The model under review builds one solid part; all positions refer to its coordinate system, in mm. A direction names the side the tool comes from. Coordinates: 2 decimals unless noted, no trailing zeros. Write each loop counter-clockwise with the first axis right and the second up, starting at its lowest first coordinate (ties: lowest second). Pieces come first, ordered by that corner, then holes.
1) Machinability: for faces 5 (the flat face through (137, 6, -5)), 6 (the flat face through (16, 0, -60)), which of the approach directions +Z, -Z, +X, -X, +Y, -Y give a long, thin tool a straight path to every point of the face, cutting with its end or side? Answer none if there is none.
2) For line 1 (Z direction, x = 287.5, y = 3.8); line 2 (Z direction, x = 385.5, y = 3.8); line 3 (X direction, y = -1, z = -129.5), list the stretches that pass through material, from the lowest coordinate up.
3) Add section C-C, the plane z = -29. State the section outline as (x, y) points.
4) Mouldability with a two-part tool opening along X and no side actions: class faces 1 (the flat face through (0, -2, -81)), 2 (the flat face through (390.8, -2, -81)), 3 (the cylindrical face through (10.12, -10.86, -108)), 4 (the cylindrical face through (380.757, -0.487, -9.349)) as released by +X, released by -X, zero draft, split by the parting line, or undercut.
5) For P1, Ø3, axis at x = 195.41, z = -129.5, coming from the -Y side; P2, Ø6, axis at x = 197, z = -15, coming from the -Y side; P3, Ø4, axis at x = 242.5, y = -9.5, coming from the -Z side, all flat-tipped, find the tip position at first contact; note any pin that passes through.
6) Add section B-B, the plane z = -78. State the section outline as (x, y) points, then the cut area to 3 significant figures.
7) Add section A-A, the plane x = 365. State the section outline as (y, z) points.
from build123d import *

# Parameters (mm, degrees)
SKETCH1_W               = 390.8
SKETCH1_H               = 133.8
BOSS_EXTRUDE1_DEPTH     = 6
SKETCH2_W               = 370.8
SKETCH2_H               = 125.6
CUT_EXTRUDE1_DEPTH      = 4
BOSS_EXTRUDE3_DEPTH     = 390.8
BOSS_EXTRUDE4_DEPTH     = 4
CUT_EXTRUDE6_DEPTH      = 414.309625425
CUT_EXTRUDE6_DEPTH_BACK = 414.309625425
SKETCH15_R              = 5
CUT_EXTRUDE8_DEPTH      = 1
SKETCH16_W              = 12.5
SKETCH16_H              = 19.4
CUT_EXTRUDE9_DEPTH      = 6
SKETCH17_W              = 390.8
SKETCH17_H              = 133.8
SKETCH17_W_2            = 386.8
SKETCH17_H_2            = 129.8
CUT_EXTRUDE10_DEPTH     = 1.7
SKETCH18_W              = 370.8
SKETCH18_H              = 4.4
BOSS_EXTRUDE5_DEPTH     = 4
M2_CLEARANCE_HOLE1_D    = 2.4
CUT_EXTRUDE7_START      = -4
SKETCH13_R              = 2.5
CUT_EXTRUDE7_DEPTH      = 410.484592101
CUT_EXTRUDE11_START     = -5
SKETCH19_R              = 2.5
CUT_EXTRUDE11_DEPTH     = 409.484592101
SKETCH20_W              = 12
SKETCH20_H              = 4
CUT_EXTRUDE12_DEPTH     = 10
FILLET1_R               = 4
FILLET2_R               = 4


# Read off the part's stored shape, not the designer's step: Boss-Extrude3
with BuildPart() as part:
    # Sketch1 → Boss-Extrude1 (new body)
    with BuildSketch(Plane(origin=(0, 0, 0), x_dir=(1, 0, 0), z_dir=(0, 1, 0))):
        with Locations((195.4, 66.9)):
            Rectangle(SKETCH1_W, SKETCH1_H)
    extrude(amount=BOSS_EXTRUDE1_DEPTH)

    # Sketch2 → Cut-Extrude1 (cut)
    with BuildSketch(Plane(origin=(0, 6, 0), x_dir=(1, 0, 0), z_dir=(0, 1, 0))):
        with Locations((195.4, 68.4)):
            Rectangle(SKETCH2_W, SKETCH2_H)
    extrude(amount=-CUT_EXTRUDE1_DEPTH, mode=Mode.SUBTRACT)

    # Boss-Extrude3 outline → Boss-Extrude3 (add)
    with BuildSketch(Plane.YZ):
        Polygon((-14.062946679, -133.8), (0, -133.8), (0, 0), align=None)
    extrude(amount=BOSS_EXTRUDE3_DEPTH)

    # Sketch10 → Boss-Extrude4 (add)
    with BuildSketch(Plane(origin=(0, 2, 0), x_dir=(1, 0, 0), z_dir=(0, 1, 0))):
        with BuildLine():
            ThreePointArc((290.5, 5.6), (287.5, 8.6), (284.5, 5.6))
            Line((284.5, 5.6), (290.5, 5.6))
        make_face()
        with BuildLine():
            Line((290.5, 5.6), (284.5, 5.6))
            ThreePointArc((284.5, 5.6), (287.5, 2.6), (290.5, 5.6))
        make_face()
        with BuildLine():
            Line((99.5, 5.6), (105.5, 5.6))
            ThreePointArc((105.5, 5.6), (102.5, 8.6), (99.5, 5.6))
        make_face()
        with BuildLine():
            ThreePointArc((99.5, 5.6), (102.5, 2.6), (105.5, 5.6))
            Line((105.5, 5.6), (99.5, 5.6))
        make_face()
    extrude(amount=BOSS_EXTRUDE4_DEPTH)

    # Sketch12 → Cut-Extrude6 (cut, two sides: drawn at the far end of the back side and taken through both)
    with BuildSketch(Plane.ZY.offset(-CUT_EXTRUDE6_DEPTH_BACK)):
        Polygon((-133.8, -14.062946679), (-118.975297196, -12.504807627), (-133.8, -0.5), align=None)
    extrude(amount=CUT_EXTRUDE6_DEPTH + CUT_EXTRUDE6_DEPTH_BACK, mode=Mode.SUBTRACT)

    # Sketch15 → Cut-Extrude8 (cut)
    with BuildSketch(Plane(origin=(0, 0, 0), x_dir=(1, 0, 0), z_dir=(0, -0.9945218953682742, 0.10452846326764666))):
        with Locations(Location((15, -109.630646394, 0), (0, 0, 270))):
            Circle(SKETCH15_R)
        with Locations(Location((375.8, -109.630646394, 0), (0, 0, 270))):
            Circle(SKETCH15_R)
        with Locations(Location((15, -10, 0), (0, 0, 270))):
            Circle(SKETCH15_R)
        with Locations(Location((375.8, -10, 0), (0, 0, 270))):
            Circle(SKETCH15_R)
    extrude(amount=-CUT_EXTRUDE8_DEPTH, mode=Mode.SUBTRACT)

    # Sketch16 → Cut-Extrude9 (cut)
    with BuildSketch(Plane(origin=(0, 6, 0), x_dir=(1, 0, 0), z_dir=(0, 1, 0))):
        with Locations((16.25, 59.4)):
            Rectangle(SKETCH16_W, SKETCH16_H)
    extrude(amount=-CUT_EXTRUDE9_DEPTH, mode=Mode.SUBTRACT)

    # Sketch17 → Cut-Extrude10 (cut)
    with BuildSketch(Plane(origin=(0, 6, 0), x_dir=(1, 0, 0), z_dir=(0, 1, 0))):
        with Locations((195.4, 66.9)):
            Rectangle(SKETCH17_W, SKETCH17_H)
        with Locations((195.4, 66.9)):
            Rectangle(SKETCH17_W_2, SKETCH17_H_2, mode=Mode.SUBTRACT)
    extrude(amount=-CUT_EXTRUDE10_DEPTH, mode=Mode.SUBTRACT)

    # Sketch18 → Boss-Extrude5 (add)
    with BuildSketch(Plane(origin=(0, 2, 0), x_dir=(1, 0, 0), z_dir=(0, 1, 0))):
        with Locations((195.4, 129)):
            Rectangle(SKETCH18_W, SKETCH18_H)
    extrude(amount=BOSS_EXTRUDE5_DEPTH)

    # M2 Clearance Hole1 (through all)
    with Locations(Plane(origin=(102.5, 6, -5.6), x_dir=(0, 0, 1), z_dir=(0, 1, 0))):
        with Locations((0, 0), (-39.4, -97.2), (-83.2, -97.2), (-83.2, 283), (-39.4, 283), (0, 185), (-123.9, 92.907395227), (-123.9, -24.518527842), (-123.9, 210.318527842)):
            Hole(M2_CLEARANCE_HOLE1_D / 2)

    # Sketch13 → Cut-Extrude7 (cut, through all)
    with BuildSketch(Plane(origin=(0, 6, 0), x_dir=(1, 0, 0), z_dir=(0, 1, 0)).offset(CUT_EXTRUDE7_START)):
        with Locations(Location((5.3, 45, 0), (0, 0, 270))):
            Circle(SKETCH13_R)
        with Locations(Location((5.3, 88.8, 0), (0, 0, 270))):
            Circle(SKETCH13_R)
        with Locations(Location((102.5, 5.6, 0), (0, 0, 270))):
            Circle(SKETCH13_R)
        with Locations(Location((287.5, 5.6, 0), (0, 0, 270))):
            Circle(SKETCH13_R)
        with Locations(Location((385.5, 45, 0), (0, 0, 270))):
            Circle(SKETCH13_R)
        with Locations(Location((385.5, 88.8, 0), (0, 0, 270))):
            Circle(SKETCH13_R)
    extrude(amount=-CUT_EXTRUDE7_DEPTH, mode=Mode.SUBTRACT)

    # Sketch19 → Cut-Extrude11 (cut, through all)
    with BuildSketch(Plane(origin=(0, 6, 0), x_dir=(1, 0, 0), z_dir=(0, 1, 0)).offset(CUT_EXTRUDE11_START)):
        with Locations(Location((77.981472158, 129.5, 0), (0, 0, 270))):
            Circle(SKETCH19_R)
        with Locations(Location((195.407395227, 129.5, 0), (0, 0, 270))):
            Circle(SKETCH19_R)
        with Locations(Location((312.818527842, 129.5, 0), (0, 0, 270))):
            Circle(SKETCH19_R)
    extrude(amount=-CUT_EXTRUDE11_DEPTH, mode=Mode.SUBTRACT)

    # Sketch20 → Cut-Extrude12 (cut)
    with BuildSketch(Plane(origin=(0, 0, -133.8), x_dir=(-1, 0, 0), z_dir=(0, 0, -1))):
        with Locations((-34.3, 4)):
            Rectangle(SKETCH20_W, SKETCH20_H)
    extrude(amount=-CUT_EXTRUDE12_DEPTH, mode=Mode.SUBTRACT)

    # Fillet1
    fillet1_edges = [part.edges().sort_by_distance(p)[0] for p in [
        (2, 5.15, -131.8),
        (2, 5.15, -2),
        (388.8, 5.15, -2),
        (388.8, 5.15, -131.8),
        (380.8, 4, -126.8),
        (10, 4, -126.8),
        (10, 4, -5.6),
        (380.8, 4, -5.6),
        (10, 1, -49.7),
        (10, 1, -69.1),
        (22.5, 1, -69.1),
        (22.5, 1, -49.7),
    ]]
    fillet(fillet1_edges, radius=FILLET1_R)

    # Fillet2
    fillet2_edges = [part.edges().sort_by_distance(p)[0] for p in [
        (290.5, 4, -5.6),
        (284.5, 4, -5.6),
        (105.5, 4, -5.6),
        (99.5, 4, -5.6),
    ]]
    fillet(fillet2_edges, radius=FILLET2_R)


solid = part.part
Geometry results:
1. face 5: +Z, -Z, +X, -X, +Y
1. face 6: +Y
2. line 1: z = -133.8 to -126.8, -8.6 to -6.8, -4.4 to 0
2. line 2: z = -133.8 to -90, -87.6 to -46.2, -43.8 to 0
2. line 3: x = 0 to 75.48, 80.48 to 192.91, 197.91 to 310.32, 315.32 to 390.8
3. outline: (0, -3.05) - (390.8, -3.05) - (390.8, 4.3) - (388.8, 4.3) - (388.8, 6) - (380.8, 6) - (380.8, 2) - (10, 2) - (10, 6) - (2, 6) - (2, 4.3) - (0, 4.3) - close
4. face 1: released by -X
4. face 2: released by +X
4. face 3: undercut
4. face 4: undercut
5. P1: stops at y = 1
5. P2: stops at y = -1.89
5. P3: stops at z = -125.16
6. outline: (0, -8.2) - (390.8, -8.2) - (390.8, 4.3) - (388.8, 4.3) - (388.8, 6) - (380.8, 6) - (380.8, 2) - (10, 2) - (10, 6) - (2, 6) - (2, 4.3) - (0, 4.3) - close
6. area: 4,060 mm2
7. outline: (-12.5, -118.98) - (-0.5, -133.8) - (4.3, -133.8) - (4.3, -131.8) - (6, -131.8) - (6, -126.8) - (2, -126.8) - (2, -5.6) - (6, -5.6) - (6, -2) - (4.3, -2) - (4.3, 0) - (0, 0) - close
